Autodesk Inventor part; units mm, degrees
ref_plane "YZ Plane" through (0, 0, 0) normal (1, 0, 0) x (0, 1, 0)
ref_plane "XZ Plane" through (0, 0, 0) normal (0, 1, 0) x (-1, 0, 0)
ref_plane "XY Plane" through (0, 0, 0) normal (0, 0, 1) x (1, 0, 0)
sketch "Sketch1" plane through (0, 0, 0) normal (0, 1, 0) x (-1, 0, 0)
  line L0 (0, 0) -> (350, 0)
  line L1 (400, 50) -> (400, 80)
  line L2 (350, 130) -> (0, 130)
  arc A0 (350, 0) -> (400, 50) centre (350, 50) ccw
  arc A1 (400, 80) -> (350, 130) centre (350, 80) ccw
  point P0 (400, 0)
  point P1 (400, 130)
  dimension "d7" = 400
  dimension "d8" = 130
  dimension "d9" = 400
  dimension "d10" = 50
sketch "Sketch2" plane through (0, 0, 0) normal (1, 0, 0) x (0, 1, 0)
  circle A0 centre (0, 0) radius 12.7
  dimension "d11" = 25.4
sweep "Sweep1" add profiles "Sketch2" path "Sketch1"
sketch "Sketch3" plane through (0, 0, 0) normal (0, 0, 1) x (1, 0, 0)
  line L0 (0, 0) -> (-30, 0)
  circle A0 centre (-30, 0) radius 6
  dimension "d14" = 30
  dimension "d15" = 12
extrude "Extrusion1" cut sketch "Sketch3" along normal through all both and the other way through all
properties part number "GARFO"
Geometry: final body of the model. Coordinates: model frame, mm. A direction names the side the tool comes from. Coordinates: 2 decimals unless noted, no trailing zeros. Write each loop counter-clockwise with the first axis right and the second up, starting at its lowest first coordinate (ties: lowest second). Pieces come first, ordered by that corner, then holes. Notation, with made-up numbers: M 12,14 L 65,14 A11 cw 65,18 Z; hole C -4,-2.5 d7. An arc over 180 degrees is marked long. Answer as CSV lines item,"result". Start each with the question number.
Q1. Cut plane A-A on y = 0. Return the cut outline in (x, z), then the cut area to 3 significant figures.
Q2. Cut plane C-C on x = -195. Return the cut outline in (y, z).
Q3. Cut plane D-D on z = 65.5. Return the cut outline in (x, y).
Q4. Line query: line 1 (Z direction, x = -297.5, y = 0); line 2 (Y direction, x = -30, z = 132.25); line 3 (Z direction, x = -141.5, y = -10.5). Output: solid intervals per line, ascending. Write a range as from..to.
Q5. Cut plane B-B on x = -30. Return the cut outline in (y, z).
Q6. Mould query, pull axis X, two halves, no side actions, for faces 4 (the cylindrical face through (-172.55, -2.75, 117.6)), 5 (the cylindrical face through (-24.46, -2.3, 0.18)), 6 (the flat face through (0, 0, 0)). Classes: released by +X, released by -X, zero draft, split by the parting line, or undercut.
Q7. Pin query (flat end, axial travel): P1, Ø1, axis at y = 8.5, z = 55.5, coming from the +X side; P2, Ø1.5, axis at y = -1.5, z = 97.5, coming from the -X side; P3, Ø1.5, axis at x = -95.5, y = -4, coming from the -Z side. Return the tip coordinate at first contact, or that it passes through.
Q8. Reachability of faces 1 (the cylindrical face through (-177.45, -2.75, 12.4)), 2 (the cylindrical face through (-412.592, -1.653, 65.21)), 3 (the flat face through (0, 0, 130)) from +Z, -Z, +X, -X, +Y, -Y: full face, straight path, thin tool, end or side. Return the list, or none.
Findings below:
1,outline,"M -412.7,50 A62.7 ccw -350,-12.7 L -36,-12.7 L -36,12.7 L -350,12.7 A37.3 cw -387.3,50 L -387.3,80 A37.3 cw -350,117.3 L -36,117.3 L -36,142.7 L -350,142.7 A62.7 ccw -412.7,80 Z; M -24,-12.7 L 0,-12.7 L 0,12.7 L -24,12.7 Z; M -24,117.3 L 0,117.3 L 0,142.7 L -24,142.7 Z"
1,area,"21,900 mm2"
2,outline,"C 0,0 d25.4; C 0,130 d25.4"
3,outline,"C -400,0 d25.4"
4,line 1,"z = -12.7..12.7, 117.3..142.7"
4,line 2,"y = -12.5..-6, 6..12.5"
4,line 3,"z = -7.14..7.14, 122.86..137.14"
5,outline,"M -6,-11.19 L -6,11.19 A12.7 ccw Z; M -6,118.81 L -6,141.19 A12.7 ccw Z; M 6,-11.19 A12.7 ccw 6,11.19 Z; M 6,118.81 A12.7 ccw 6,141.19 Z"
6,face 4,"zero draft"
6,face 5,"undercut"
6,face 6,"released by +X"
7,P1,"stops at x = -390.14"
7,P2,"stops at x = -410.35"
7,P3,"stops at z = -12.28"
8,face 1,"+X"
8,face 2,"none"
8,face 3,"+Z, -Z, +X, +Y, -Y"
